from build123d import *

# Parameters (mm, degrees)
F0_W     = 100
F0_H     = 80
F1_DEPTH = 15
F3_DEPTH = 35
F4_R     = 30
F5_DEPTH = 35
F6_SIZE  = 5
F7_R     = 15
F8_DEPTH = 40
F9_R     = 10


with BuildPart() as f1:
    # F0 (on Top) → F1 (new body)
    with BuildSketch(Plane.XY):
        with Locations((50, 40)):
            Rectangle(F0_W, F0_H)
    extrude(amount=F1_DEPTH)

    # F2 (on face) → F3 (join)
    with BuildSketch(Plane.XY.offset(15)):
        Polygon((20, 80), (0, 80), (0, 60), align=None)
    extrude(amount=F3_DEPTH)

    # F4 (on face) → F5 (join)
    with BuildSketch(Plane.XY.offset(15)):
        with Locations((50, 40)):
            Circle(F4_R)
    extrude(amount=F5_DEPTH)

    # F6
    f6_edges = [f1.edges().sort_by_distance(p)[0] for p in [
        (20, 40, 50),
    ]]
    chamfer(f6_edges, length=F6_SIZE)

    # F7 (on face) → F8 (cut)
    with BuildSketch(Plane.XY.offset(50)):
        with Locations((50, 40)):
            Circle(F7_R)
    extrude(amount=-F8_DEPTH, mode=Mode.SUBTRACT)

    # F9
    f9_edges = [f1.edges().sort_by_distance(p)[0] for p in [
        (35, 40, 10),
    ]]
    fillet(f9_edges, radius=F9_R)


solid = f1.part
For this review, take the finished solid that the model builds, in its own axes (mm). A direction names the side the tool comes from. Give positions to 0.01 mm unless a question says otherwise; leave off trailing zeros. Loops run counter-clockwise (first coordinate to the right, second up) from the corner with the lowest first, then second, coordinate; pieces in that order, holes last. Notation, with made-up numbers: M 88.5,2.25 L 134.5,2.25 A10 cw 134.5,11.25 Z; hole C 79.5,13.5 d4. An arc over 180 degrees is marked long. Answer as a JSON object with one key per item and string values. Group by question number.
Q1. Add section A-A on x = 87. Give the boundary of the cut face in (y, z).
Q2. Insertion check: P1, Ø18, axis at x = 50, y = 40, coming from the +Z side; P2, Ø6, axis at x = 47.5, z = 42.5, coming from the +Y side; P3, Ø12, axis at x = 35, z = 42, coming from the +Y side. Each pin has a flat end and moves straight along its axis. Give the tip position at first contact, or say it passes through.
Q3. Tool access review of faces 1 (the flat face through (61, 29, 50)), 2 (the flat face through (10, 70, 32)), 3 (the flat face through (50, 40, 10)): name each direction out of +Z, -Z, +X, -X, +Y, -Y from which nothing blocks a thin tool from reaching the whole face with its end or side.
Q4. Mouldability with a two-part tool opening along X and no side actions: class faces 4 (the flat face through (49, 41, 0)), 5 (the cylindrical face through (38.944, 50.138, 35.21)), 6 (the flat face through (0, 49, 14)), 7 (the conical face through (73.318, 30.332, 49.757)) as +X half, -X half, draft (parallel to the pull), parting line (faces both ways), or undercut.
Q5. For probe 1 along Y at (x, z) = (50, 28.25); probe 2 along Z at (x, y) = (38, 10); probe 3 along Y at (x, z) = (43, 31.5), list the stretches that pass through material, from the lowest coordinate up. Write a range as [from, to].
Checked values:
{
 "1": {"outline": "M 0,0 L 80,0 L 80,15 L 0,15 Z"},
 "2": {"P1": "z = 10.83", "P2": "y = 70", "P3": "y = 68.62"},
 "3": {"face 1": "+Z, +X, -X, +Y, -Y", "face 2": "+Z, -Y", "face 3": "+Z"},
 "4": {"face 4": "draft", "face 5": "undercut", "face 6": "-X half", "face 7": "undercut"},
 "5": {"probe 1": "[10, 25], [55, 70]", "probe 2": "[0, 15]", "probe 3": "[10.83, 26.73], [53.27, 69.17]"}
}
